from build123d import *

# Parameters (mm, degrees)
F0_W     = 106.33587
F0_H     = 63.491806
F1_DEPTH = 25.4
F2_R     = 6.35
F2_R_2   = 6.349997
F2_R_3   = 6.313875
F3_DEPTH = 25.4
F4_R     = 15.282294
F5_DEPTH = 38.1


with BuildPart() as f1:
    # F0 (on Top) → F1 (new body)
    with BuildSketch(Plane.XY):
        Rectangle(F0_W, F0_H)
    extrude(amount=F1_DEPTH)

    # F2 (on face) → F3 (cut)
    with BuildSketch(Plane.XY.offset(25.4)):
        with Locations((-44.392645, 23.228709)):
            Circle(F2_R)
        with Locations((-44.13455, -22.45442)):
            Circle(F2_R_2)
        with Locations((43.360256, 23.744902)):
            Circle(F2_R_3)
        with Locations((42.844065, -22.712516)):
            Circle(F2_R_3)
    extrude(amount=-F3_DEPTH, mode=Mode.SUBTRACT)

    # F4 (on face) → F5 (join)
    with BuildSketch(Plane.XY.offset(25.4)):
        Circle(F4_R)
    extrude(amount=F5_DEPTH)


solid = f1.part
Source: CAD feature listing. Evaluate the final solid. Frame: model axes, mm. A direction names the side the tool comes from. Round coordinates to 2 decimals unless told otherwise and drop trailing zeros. Loops run counter-clockwise (first coordinate to the right, second up) from the corner with the lowest first, then second, coordinate; pieces in that order, holes last. Notation, with made-up numbers: (52.25, 70.25) - (62.25, 70.25) arc R33 ccw to (62.25, 108.25) - close; hole circle Ø3 at (65, 67). An arc over 180 degrees is marked (long way). Write item = value, one per line. Start each with the question number.
Item 1: Mould query, pull axis Y, two halves, no side actions, for faces 3 (the face through (-44.96, -16.16, 12.88)), 4 (the face through (-1, 31.746, 13)), 5 (the face through (-1, -31.746, 13)). Classes: released by +Y, released by -Y, zero draft, split by the parting line, or undercut.
Item 2: Material intervals for line 1 (Y direction, x = 48.5, z = 4.5); line 2 (X direction, y = -18.5, z = 20); line 3 (Y direction, x = -41, z = 5.5), sorted ascending.
Item 3: Section query A-A on x = 0. Output: boundary loops of the cut face in (y, z), plus the area to 3 significant figures.
Item 4: Section query B-B on x = 45. Output: boundary loops of the cut face in (y, z), plus the area to 3 significant figures.
Item 5: First-contact query: pin 1 Ø10 at (x, y) = (-44.39, 23.23) entering from +Z; pin 2 Ø16.5 at (x, y) = (43.36, 23.74) entering from +Z; pin 3 Ø12 at (y, z) = (-8.5, 52) entering from -X. Flat tips, straight axial feed; report the tip coordinate or a pass-through.
Item 6: Section query D-D on z = 5. Output: boundary loops of the cut face in (x, y).
Item 7: Reachability of faces 1 (the face through (41.475, -28.876, 12.878)), 2 (the face through (-12.128, -9.299, 44.183)) from +Z, -Z, +X, -X, +Y, -Y: full face, straight path, thin tool, end or side. Return the list, or none.
Item 8: Section query C-C on y = 0. Output: boundary loops of the cut face in (x, z).
Results list:
q1.face_3 = undercut
q1.face_4 = released by +Y
q1.face_5 = released by -Y
q2.line_1 = -31.75 to -25.52, -19.91 to 20.08, 27.41 to 31.75
q2.line_2 = -53.17 to -49.1, -39.17 to 38.14, 47.55 to 53.17
q2.line_3 = -31.75 to -27.98, -16.93 to 17.86, 28.6 to 31.75
q3.outline = (-31.75, 0) - (31.75, 0) - (31.75, 25.4) - (15.28, 25.4) - (15.28, 63.5) - (-15.28, 63.5) - (-15.28, 25.4) - (-31.75, 25.4) - close
q3.area = 2,780 mm²
q4.outline = (-31.75, 0) - (-28.65, 0) - (-28.65, 25.4) - (-31.75, 25.4) - close; (-16.78, 0) - (17.65, 0) - (17.65, 25.4) - (-16.78, 25.4) - close; (29.84, 0) - (31.75, 0) - (31.75, 25.4) - (29.84, 25.4) - close
q4.area = 1,000 mm²
q5.pin_1 = through
q5.pin_2 = 25.4
q5.pin_3 = -15.08
q6.outline = (-53.17, -31.75) - (53.17, -31.75) - (53.17, 31.75) - (-53.17, 31.75) - close; hole circle Ø12.7 at (-44.39, 23.23); hole circle Ø12.7 at (-44.13, -22.45); hole circle Ø12.63 at (42.84, -22.71); hole circle Ø12.63 at (43.36, 23.74)
q7.face_1 = +Z, -Z
q7.face_2 = +Z
q8.outline = (-53.17, 0) - (53.17, 0) - (53.17, 25.4) - (15.28, 25.4) - (15.28, 63.5) - (-15.28, 63.5) - (-15.28, 25.4) - (-53.17, 25.4) - close
